Can you work these out from the drawing? Everything is in mm from the part's minimum corner. Coordinates: 2 decimals unless noted, no trailing zeros. Order: outer loops, then holes, each group sorted by start corner. A loop starts at its lowest first (then second) coordinate and runs counter-clockwise, first axis right, second up. Notation, with made-up numbers: (42, -39.5) -> (72, -39.5) arc R38 cw to (72, -1.5) -> close; hole circle Ø4 at (-36, 28). An arc over 180 degrees is marked (long way). Return JSON: item names as keys, results as strings. Group by question number.
1) If we section it at B-B, the plane x = 115: Please give me the cut outline in (y, z).
2) If we section it at A-A, the plane z = 5: Please give me the cut outline in (x, y).
3) If I drill on probe 1 along X at (y, z) = (1.85, 5); probe 2 along Z at (x, y) = (5, 3.85); probe 3 along X at (y, z) = (2.5, 6), over which ranges is the centre line in solid material (lowest first)? Write a range as from..to.
4) For pin 1 (2 mm diameter, centred on x = 27.5, y = 4, fed in from -Z); pin 2 (2.5 mm diameter, centred on x = 5, z = 75, fed in from +Y), each with a flat end and sliding along its axis, tell me the tip position at first contact or that it passes through.
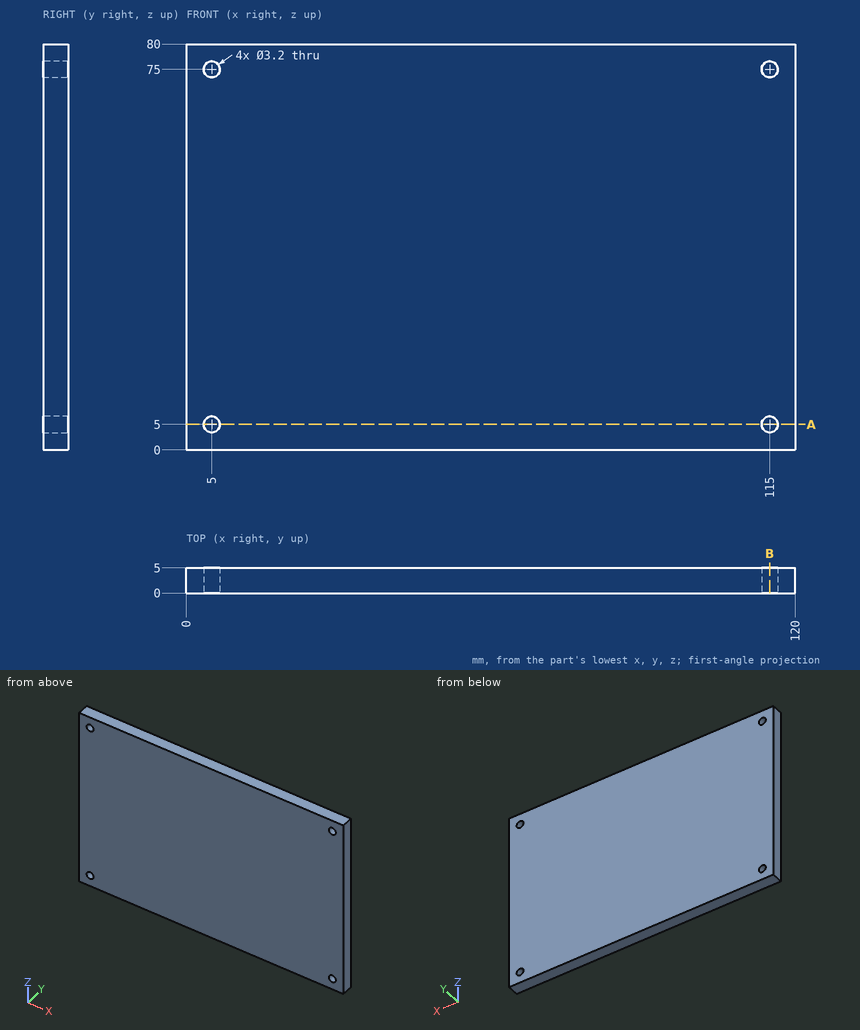
Result sheet:
{
 "1": {"outline": "(0, 0) -> (5, 0) -> (5, 3.4) -> (0, 3.4) -> close; (0, 6.6) -> (5, 6.6) -> (5, 73.4) -> (0, 73.4) -> close; (0, 76.6) -> (5, 76.6) -> (5, 80) -> (0, 80) -> close"},
 "2": {"outline": "(0, 0) -> (3.4, 0) -> (3.4, 5) -> (0, 5) -> close; (6.6, 0) -> (113.4, 0) -> (113.4, 5) -> (6.6, 5) -> close; (116.6, 0) -> (120, 0) -> (120, 5) -> (116.6, 5) -> close"},
 "3": {"probe 1": "x = 0..3.4, 6.6..113.4, 116.6..120", "probe 2": "z = 0..3.4, 6.6..73.4, 76.6..80", "probe 3": "x = 0..3.75, 6.25..113.75, 116.25..120"},
 "4": {"pin 1": "stops at z = 0", "pin 2": "passes through"}
}
